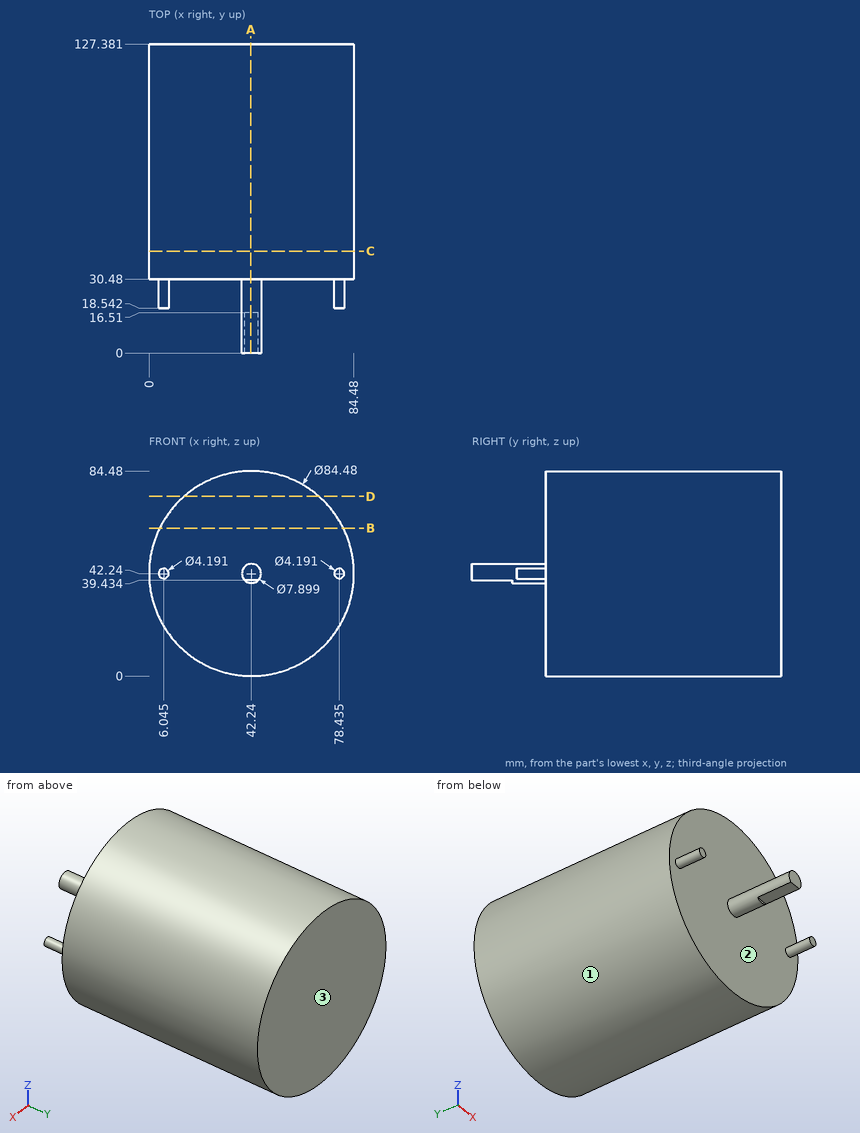
Can you work these out from the drawing? Everything is in mm from the part's minimum corner. Coordinates: 2 decimals unless noted, no trailing zeros. Write each loop counter-clockwise with the first axis right and the second up, starting at its lowest first coordinate (ties: lowest second). Pieces come first, ordered by that corner, then holes. Notation, with made-up numbers: (17.25, -20.5) - (47.25, -20.5) arc R29 cw to (47.25, 12.5) - close; hole circle Ø11 at (-37, -8.75). An arc over 180 degrees is marked (long way). One line per item, written item: value.
1) Suppose I cut it at B-B on z = 61. Write out the boundary of the cut face in (x, y) (1 decimal).
Model answer:
outline: (4.4, 30.5) - (80.1, 30.5) - (80.1, 127.4) - (4.4, 127.4) - close
2) Suppose I cut it at A-A on x = 42. Write out the boundary of the cut face in (y, z).
Model answer:
outline: (0, 39.43) - (16.51, 39.43) - (16.51, 38.3) - (30.48, 38.3) - (30.48, 0) - (127.38, 0) - (127.38, 84.48) - (30.48, 84.48) - (30.48, 46.18) - (0, 46.18) - close
3) Suppose I cut it at C-C on y = 42. Write out the boundary of the cut face in (x, z), and give its area (3 significant figures).
Model answer:
outline: circle Ø84.48 at (42.24, 42.24)
area: 5,610 mm²
4) We'd pull the mould along Y, two halves only. Please class the marked faces 1, 2 and 3: pulls with the +Y half, pulls with the -Y half, needs draft (parallel to the pull), parting line crosses it, or undercut.
Model answer:
face 1: needs draft
face 2: pulls with the -Y half
face 3: pulls with the +Y half
5) I need wall thicknesses on line 1 along Y through (x, z) = (37, 20); line 2 along Z through (x, y) = (30.5, 104) (1 decimal); line 3 along X through (y, z) = (55.5, 10). Which ranges of each line are inside material? Lowest first, please.
Model answer:
line 1: y = 30.48 to 127.38
line 2: z = 1.7 to 82.8
line 3: x = 14.95 to 69.53
6) Suppose I cut it at D-D on z = 74. Write out the boundary of the cut face in (x, y).
Model answer:
outline: (14.39, 30.48) - (70.09, 30.48) - (70.09, 127.38) - (14.39, 127.38) - close
7) I'm going to push flat-ended pins straight in: P1, Ø12, axis at y = 88, z = 72.5, coming from the -X side; P2, Ø1.7, axis at x = 42, y = 10, coming from the -Z side; P3, Ø4.5, axis at x = 78.5, z = 41.5, coming from the -Y side. Where does each tip first touch, or does it pass through?
Model answer:
P1: stops at x = 7.66
P2: stops at z = 39.43
P3: stops at y = 18.54
